```python
from build123d import *

# Parameters (mm, degrees)
BOSS_EXTRUDE1_DEPTH   = 13
F_6_0MM_DOWEL_HOLE1_D = 6


with BuildPart() as part:
    # Sketch1 → Boss-Extrude1 (new body)
    with BuildSketch(Plane(origin=(0, 0, 0), x_dir=(1, 0, 0), z_dir=(0, 1, 0))):
        with BuildLine():
            Line((5, 0), (15, 0))
            ThreePointArc((15, 0), (18.535533906, 1.464466094), (20, 5))
            Line((20, 5), (20, 55))
            ThreePointArc((20, 55), (18.535533906, 58.535533906), (15, 60))
            Line((15, 60), (5, 60))
            ThreePointArc((5, 60), (1.464466094, 58.535533906), (0, 55))
            Line((0, 55), (0, 5))
            ThreePointArc((0, 5), (1.464466094, 1.464466094), (5, 0))
        make_face()
    extrude(amount=BOSS_EXTRUDE1_DEPTH)

    # Ø6.0mm Dowel Hole1 (through all)
    with Locations(Plane(origin=(0, 13, 0), x_dir=(1, 0, 0), z_dir=(0, 1, 0))):
        with Locations((10, 12), (10, 48)):
            Hole(F_6_0MM_DOWEL_HOLE1_D / 2)


solid = part.part
```
Could you check a few things on this model? Use its own coordinates, in mm. Round coordinates to 2 decimals unless told otherwise and drop trailing zeros. Write each loop counter-clockwise with the first axis right and the second up, starting at its lowest first coordinate (ties: lowest second). Pieces come first, ordered by that corner, then holes. Notation, with made-up numbers: M -1.75,-9.75 L 4.25,-9.75 A24 ccw 4.25,10.25 Z; hole C -24.5,-22.5 d1. An arc over 180 degrees is marked long. Write each question's results on one line, items separated by ' | '. Start each with the question number.
1. I need wall thicknesses on L1, parallel to Z at x = 10, y = 10; L2, parallel to X at y = 4.75, z = -12; L3, parallel to X at y = 8.75, z = -10.5. Which ranges of each line are inside material? Lowest first, please. Write a range as from..to.
2. Imagine slicing it at D-D on x = 2. List the corners of the cut face in (y, z) for me, and give its area (3 significant figures).
3. Imagine slicing it at C-C on y = 2. List the corners of the cut face in (x, z) for me, and give its area (3 significant figures).
4. Imagine slicing it at A-A on x = 10. List the corners of the cut face in (y, z) for me.
5. Thinking about a two-plate mould opening in X: for faces 1 (the face through (10, 6, -51)), 2 (the face through (2, 6, -59)), 3 (the face through (10, 0, -30)), which applies, +X half, -X half, draft (parallel to the pull), parting line (faces both ways), or undercut?
6. Imagine slicing it at B-B on z = -48. List the corners of the cut face in (x, y) for me, and give its area (3 significant figures).
Result sheet:
1) L1: z = -60..-51, -45..-15, -9..0 | L2: x = 0..7, 13..20 | L3: x = 0..7.4, 12.6..20
2) outline: M 0,-59 L 13,-59 L 13,-1 L 0,-1 Z | area: 754 mm^2
3) outline: M 0,-55 A5 ccw 5,-60 L 15,-60 A5 ccw 20,-55 L 20,-5 A5 ccw 15,0 L 5,0 A5 ccw 0,-5 Z; hole C 10,-48 d6; hole C 10,-12 d6 | area: 1,120 mm^2
4) outline: M 0,-60 L 13,-60 L 13,-51 L 0,-51 Z; M 0,-45 L 13,-45 L 13,-15 L 0,-15 Z; M 0,-9 L 13,-9 L 13,0 L 0,0 Z
5) face 1: undercut | face 2: -X half | face 3: draft
6) outline: M 0,0 L 7,0 L 7,13 L 0,13 Z; M 13,0 L 20,0 L 20,13 L 13,13 Z | area: 182 mm^2
